For this review, take the finished solid that the model builds, in its own axes (mm). A direction names the side the tool comes from. Give positions to 0.01 mm unless a question says otherwise; leave off trailing zeros. Order: outer loops, then holes, each group sorted by start corner. A loop starts at its lowest first (then second) coordinate and runs counter-clockwise, first axis right, second up. Notation, with made-up numbers: (-20, 80) -> (-10, 80) arc R19 ccw to (-10, 105) -> close; hole circle Ø11 at (78, -27). An arc over 180 degrees is marked (long way). Return JSON: item names as keys, results as strings. Group by question number.
1) Add section D-D (y = 18). Give the boundary of the cut face in (x, z).
2) To check wall thickness, follow line 1 along Y through (x, z) = (16, -233); line 2 along X through (y, z) = (198.5, 115); line 3 along Y through (x, z) = (106, -48.5). State the ranges of each line that lie inside material, in increasing order.
3) Add section C-C (z = -139). Give the boundary of the cut face in (x, y), then the cut area to 3 significant figures.
4) Insertion check: P1, Ø0.6, axis at x = 153, y = -1, coming from the +Z side; P2, Ø4, axis at y = 23, z = -31, coming from the -X side; P3, Ø1.6, axis at y = -1, z = -201, coming from the -X side; P4, Ø1, axis at x = -156, z = 45.5, coming from the +Y side. Each pin has a flat end and moves straight along its axis. Give the tip position at first contact, or say it passes through.
5) Add section A-A (z = 0). Give the boundary of the cut face in (x, y), then the cut area to 3 significant figures.
6) The part is to be moulded in two halves that separate along X. For faces 1 (the face through (-1, 109, -240)), 2 (the face through (82.6, 2.5, 262.3)), 3 (the face through (146.647, -2.986, 137.229)), say which applies: released by +X, released by -X, zero draft, split by the parting line, or undercut.
7) Add section B-B (x = 0). Give the boundary of the cut face in (y, z), then the cut area to 3 significant figures.
8) For faces 4 (the face through (82, 180, -3)), 5 (the face through (-153.69, -2.99, 131.32)), 6 (the face through (-1, 109, 240)), 7 (the face through (1, 214.5, 3)), 8 (the face through (-95, 91, 3)), list the 3-axis set-ups (+Z, -Z, +X, -X, +Y, -Y) from which the entire face can be reached by the end or side of a thin tool; tool diameter is ignored.
from build123d import *

# Parameters (mm, degrees)
SKETCH_1_R      = 275
SKETCH_1_W      = 90
SKETCH_1_H      = 190
EXTRUDE_1_DEPTH = 5
SKETCH_1_4_W    = 190
SKETCH_1_4_H    = 480
EXTRUDE_2_DEPTH = 180
EXTRUDE_3_DEPTH = 480
SKETCH_5_W      = 45
SKETCH_5_H      = 45
SKETCH_5_R      = 12
EXTRUDE_4_DEPTH = 2
SKETCH_5_3_R    = 12
EXTRUDE_5_DEPTH = 4


with BuildPart() as part:
    # 草图1 → 凸台-拉伸1 (new body)
    with BuildSketch(Plane(origin=(0, 0, 0), x_dir=(1, 0, 0), z_dir=(0, 1, 0))):
        with Locations(Location((0, 0, 0), (0, 0, 270))):
            Circle(SKETCH_1_R)
        with Locations((-200, 0)):
            Rectangle(SKETCH_1_W, SKETCH_1_H, mode=Mode.SUBTRACT)
        with Locations((200, 0)):
            Rectangle(SKETCH_1_W, SKETCH_1_H, mode=Mode.SUBTRACT)
    extrude(amount=EXTRUDE_1_DEPTH)

    # 草图1<4> → 凸台-拉伸2 (add)
    with BuildSketch(Plane(origin=(0, 0, 0), x_dir=(1, 0, 0), z_dir=(0, 1, 0))):
        Rectangle(SKETCH_1_4_W, SKETCH_1_4_H)
    extrude(amount=EXTRUDE_2_DEPTH)

    # 草图2 → 凸台-拉伸3 (add)
    with BuildSketch(Plane.XY.offset(240)):
        Polygon((-68.5, 214.5), (-68.5, 181.5), (-68.5, 180), (-70, 180), (-70, 216), (70, 216), (70, 180), (68.5, 180), (68.5, 181.5), (68.5, 214.5), align=None)
    extrude(amount=-EXTRUDE_3_DEPTH)

    # 草图5 → 凸台-拉伸4 (add)
    # profile 1 of 3: a face of its own
    with BuildSketch(Plane.XZ):
        with Locations((-157.292912236, 142.766592664)):
            Rectangle(SKETCH_5_W, SKETCH_5_H)
        with Locations(Location((-157.292912236, 142.766592664, 0), (0, 0, 270))):
            Circle(SKETCH_5_R, mode=Mode.SUBTRACT)
    # profile 2 of 3: a face of its own
    with BuildSketch(Plane.XZ):
        with Locations((157.292912236, 142.766592664)):
            Rectangle(SKETCH_5_W, SKETCH_5_H)
        with Locations(Location((157.292912236, 142.766592664, 0), (0, 0, 270))):
            Circle(SKETCH_5_R, mode=Mode.SUBTRACT)
    # profile 3 of 3: a face of its own
    with BuildSketch(Plane.XZ):
        with Locations((0, -194.549146173)):
            Rectangle(SKETCH_5_W, SKETCH_5_H)
        with Locations(Location((0, -194.549146173, 0), (0, 0, 270))):
            Circle(SKETCH_5_R, mode=Mode.SUBTRACT)
    extrude(amount=EXTRUDE_4_DEPTH)

    # 草图5<3> → 凸台-拉伸5 (add)
    with BuildSketch(Plane.XZ):
        with Locations(Location((-157.292912236, 142.766592664, 0), (0, 0, 270))):
            Circle(SKETCH_5_3_R)
        with Locations(Location((0, -194.549146173, 0), (0, 0, 270))):
            Circle(SKETCH_5_3_R)
        with Locations(Location((157.292912236, 142.766592664, 0), (0, 0, 270))):
            Circle(SKETCH_5_3_R)
    extrude(amount=EXTRUDE_5_DEPTH)


solid = part.part
Evaluation:
{
 "1": {"outline": "(-95, -240) -> (95, -240) -> (95, 240) -> (-95, 240) -> close"},
 "2": {"line 1": "0 to 180, 214.5 to 216", "line 2": "-70 to -68.5, 68.5 to 70", "line 3": "0 to 5"},
 "3": {"outline": "(-237.28, 0) -> (237.28, 0) -> (237.28, 5) -> (95, 5) -> (95, 180) -> (70, 180) -> (70, 216) -> (-70, 216) -> (-70, 180) -> (-95, 180) -> (-95, 5) -> (-237.28, 5) -> close; hole (-68.5, 180) -> (68.5, 180) -> (68.5, 214.5) -> (-68.5, 214.5) -> close", "area": "35,900 mm^2"},
 "4": {"P1": "z = 165.27", "P2": "x = -95", "P3": "x = -22.5", "P4": "through"},
 "5": {"outline": "(-275, 0) -> (-245, 0) -> (-245, 5) -> (-275, 5) -> close; (-155, 0) -> (155, 0) -> (155, 5) -> (95, 5) -> (95, 180) -> (70, 180) -> (70, 216) -> (-70, 216) -> (-70, 180) -> (-95, 180) -> (-95, 5) -> (-155, 5) -> close; (245, 0) -> (275, 0) -> (275, 5) -> (245, 5) -> close; hole (-68.5, 180) -> (68.5, 180) -> (68.5, 214.5) -> (-68.5, 214.5) -> close", "area": "35,400 mm^2"},
 "6": {"face 1": "zero draft", "face 2": "split by the parting line", "face 3": "undercut"},
 "7": {"outline": "(-4, -206.55) -> (-2, -206.55) -> (-2, -217.05) -> (0, -217.05) -> (0, -275) -> (5, -275) -> (5, -240) -> (180, -240) -> (180, 240) -> (5, 240) -> (5, 275) -> (0, 275) -> (0, -172.05) -> (-2, -172.05) -> (-2, -182.55) -> (-4, -182.55) -> close; (214.5, -240) -> (216, -240) -> (216, 240) -> (214.5, 240) -> close", "area": "87,600 mm^2"},
 "8": {"face 4": "+Z, -Z, +X, +Y", "face 5": "-Y", "face 6": "+Z, +X, -X, +Y", "face 7": "+Z, -Z", "face 8": "+Z, -Z, -X, +Y"}
}
